Geometry: final body of the model. Coordinates: model frame, mm. A direction names the side the tool comes from. Give positions to 0.01 mm unless a question says otherwise; leave off trailing zeros. Write each loop counter-clockwise with the first axis right and the second up, starting at its lowest first coordinate (ties: lowest second). Pieces come first, ordered by that corner, then holes. Notation, with made-up numbers: (-39, 80.5) -> (8, 80.5) arc R19 ccw to (8, 109.5) -> close; hole circle Ø3 at (-22, -11). An arc over 180 degrees is marked (long way). Answer as a JSON object with one key per item and string values. Group by question number.
(1) Contact query for flat-ended pins moving along their axis: pin 1 Ø8 at (x, y) = (-12.5, -12.5) entering from -Z; pin 2 Ø5 at (x, z) = (-0.5, 9.5) entering from -Y. Output: stop coordinate, or through.
(2) Section query C-C on y = -20.5. Output: boundary loops of the cut face in (x, z), plus the area to 3 significant figures.
(3) Section query B-B on y = -25. Output: boundary loops of the cut face in (x, z), plus the area to 3 significant figures.
(4) Set-up query: faces 1 (the face through (-18, -40, 7)), 2 (the face through (-17, -20, 7)). Return all of +Z, -Z, +X, -X, +Y, -Y with unobstructed straight access to the full face (end or side cutting, diameter ignored); none if empty.
(5) Draft query along X for faces 3 (the face through (-19, -19, 7)), 4 (the face through (0, 0, 7)), 5 (the face through (18, -27, 7)), 6 (the face through (17, -20, 7)). Return one class per face: +X half, -X half, draft (parallel to the pull), parting line (faces both ways), or undercut.
(6) Section query D-D on z = 3. Output: boundary loops of the cut face in (x, y).
(7) Material intervals for probe 1 along Z at (x, y) = (-18.4, -25); probe 2 along X at (y, z) = (-36.5, 7.5); probe 3 along Y at (x, z) = (-16, 7.5), sorted ascending.
(8) Section query A-A on z = 7. Output: boundary loops of the cut face in (x, y), plus the area to 3 significant figures.
from build123d import *

# Parameters (mm, degrees)
PAD_DEPTH    = 14
SKETCH001_R  = 2
POCKET_DEPTH = 38.001


with BuildPart() as part:
    # Sketch → Pad (new body)
    with BuildSketch(Plane.XY):
        Polygon((-17, -40), (-17, 0), (17, 0), (17, -40), (19, -40), (19, 2), (-19, 2), (-19, -40), align=None)
    extrude(amount=PAD_DEPTH)

    # Sketch001 (on Face5 of Pad) → Pocket (cut, through all)
    with BuildSketch(Plane.YZ.offset(19)):
        with Locations((-25, 7)):
            Circle(SKETCH001_R)
    extrude(amount=-POCKET_DEPTH, mode=Mode.SUBTRACT)


solid = part.part
Answer list:
{
 "1": {"pin 1": "through", "pin 2": "y = 0"},
 "2": {"outline": "(-19, 0) -> (-17, 0) -> (-17, 14) -> (-19, 14) -> close; (17, 0) -> (19, 0) -> (19, 14) -> (17, 14) -> close", "area": "56.0 mm2"},
 "3": {"outline": "(-19, 0) -> (-17, 0) -> (-17, 5) -> (-19, 5) -> close; (-19, 9) -> (-17, 9) -> (-17, 14) -> (-19, 14) -> close; (17, 0) -> (19, 0) -> (19, 5) -> (17, 5) -> close; (17, 9) -> (19, 9) -> (19, 14) -> (17, 14) -> close", "area": "40.0 mm2"},
 "4": {"face 1": "+Z, -Z, +X, -X, -Y", "face 2": "+Z, -Z, -Y"},
 "5": {"face 3": "-X half", "face 4": "undercut", "face 5": "draft", "face 6": "undercut"},
 "6": {"outline": "(-19, -40) -> (-17, -40) -> (-17, 0) -> (17, 0) -> (17, -40) -> (19, -40) -> (19, 2) -> (-19, 2) -> close"},
 "7": {"probe 1": "0 to 5, 9 to 14", "probe 2": "-19 to -17, 17 to 19", "probe 3": "0 to 2"},
 "8": {"outline": "(-19, -40) -> (-17, -40) -> (-17, -27) -> (-19, -27) -> close; (-19, -23) -> (-17, -23) -> (-17, 0) -> (17, 0) -> (17, -23) -> (19, -23) -> (19, 2) -> (-19, 2) -> close; (17, -40) -> (19, -40) -> (19, -27) -> (17, -27) -> close", "area": "220 mm2"}
}
